Here's how the part is built. I have some questions about the finished solid (model axes, mm). A direction names the side the tool comes from. Give positions to 0.01 mm unless a question says otherwise; leave off trailing zeros. Write each loop counter-clockwise with the first axis right and the second up, starting at its lowest first coordinate (ties: lowest second). Pieces come first, ordered by that corner, then holes. Notation, with made-up numbers: (-26.5, 23) -> (-22.5, 23) arc R25 ccw to (-22.5, 59) -> close; hole circle Ø4 at (-4.75, -37). An arc over 180 degrees is marked (long way). Put each result on its own line as item: value. Start each with the question number.
from build123d import *

# Parameters (mm, degrees)
SKETCH_1_W      = 104
SKETCH_1_H      = 64
SKETCH_1_W_2    = 98
SKETCH_1_H_2    = 58
EXTRUDE_1_DEPTH = 2
SKETCH_1_3_W    = 104
SKETCH_1_3_H    = 64
EXTRUDE_2_DEPTH = 3
SKETCH_2_W      = 2
SKETCH_2_H      = 5
SKETCH_2_W_2    = 10
SKETCH_2_H_2    = 2
EXTRUDE_3_DEPTH = 2
EXTRUDE_START   = 2
SKETCH_1_4_W    = 104
SKETCH_1_4_H    = 64
SKETCH_1_4_W_2  = 98
SKETCH_1_4_H_2  = 58
EXTRUDE_4_DEPTH = 8.5
SKETCH_3_W      = 10
SKETCH_3_H      = 2
EXTRUDE_5_DEPTH = 2
EXTRUDE_START_2 = 10.5
SKETCH_1_5_W    = 104
SKETCH_1_5_H    = 64
SKETCH_1_5_W_2  = 98
SKETCH_1_5_H_2  = 58
EXTRUDE_6_DEPTH = 2


with BuildPart() as part:
    # 草图1 → 凸台-拉伸1 (new body)
    with BuildSketch(Plane(origin=(0, 0, 0), x_dir=(1, 0, 0), z_dir=(0, 1, 0))):
        Rectangle(SKETCH_1_W, SKETCH_1_H)
        Rectangle(SKETCH_1_W_2, SKETCH_1_H_2, mode=Mode.SUBTRACT)
    extrude(amount=EXTRUDE_1_DEPTH)

    # 草图1<3> → 凸台-拉伸2 (add)
    with BuildSketch(Plane(origin=(0, 0, 0), x_dir=(1, 0, 0), z_dir=(0, 1, 0))):
        Rectangle(SKETCH_1_3_W, SKETCH_1_3_H)
    extrude(amount=-EXTRUDE_2_DEPTH)

    # 草图2 → 凸台-拉伸3 (add)
    with BuildSketch(Plane(origin=(0, 0, 0), x_dir=(1, 0, 0), z_dir=(0, 1, 0))):
        with Locations((-48, 0)):
            Rectangle(SKETCH_2_W, SKETCH_2_H)
        with Locations((48, 0)):
            Rectangle(SKETCH_2_W, SKETCH_2_H)
        with Locations((0, 28)):
            Rectangle(SKETCH_2_W_2, SKETCH_2_H_2)
        with Locations((0, -28)):
            Rectangle(SKETCH_2_W_2, SKETCH_2_H_2)
    extrude(amount=EXTRUDE_3_DEPTH)

    # 草图1<4> → 凸台-拉伸4 (add)
    with BuildSketch(Plane(origin=(0, 0, 0), x_dir=(1, 0, 0), z_dir=(0, 1, 0)).offset(EXTRUDE_START)):
        Rectangle(SKETCH_1_4_W, SKETCH_1_4_H)
        Rectangle(SKETCH_1_4_W_2, SKETCH_1_4_H_2, mode=Mode.SUBTRACT)
    extrude(amount=EXTRUDE_4_DEPTH)

    # 草图3 → 凸台-拉伸5 (add)
    with BuildSketch(Plane(origin=(0, 10.5, 0), x_dir=(1, 0, 0), z_dir=(0, 1, 0))):
        with Locations((40, -28)):
            Rectangle(SKETCH_3_W, SKETCH_3_H)
        with Locations((-40, -28)):
            Rectangle(SKETCH_3_W, SKETCH_3_H)
        with Locations((40, 28)):
            Rectangle(SKETCH_3_W, SKETCH_3_H)
        with Locations((-40, 28)):
            Rectangle(SKETCH_3_W, SKETCH_3_H)
    extrude(amount=-EXTRUDE_5_DEPTH)

    # 草图1<5> → 凸台-拉伸6 (add)
    with BuildSketch(Plane(origin=(0, 0, 0), x_dir=(1, 0, 0), z_dir=(0, 1, 0)).offset(EXTRUDE_START_2)):
        Rectangle(SKETCH_1_5_W, SKETCH_1_5_H)
        Rectangle(SKETCH_1_5_W_2, SKETCH_1_5_H_2, mode=Mode.SUBTRACT)
    extrude(amount=EXTRUDE_6_DEPTH)


solid = part.part
1) Thinking about a two-plate mould opening in Y: for faces 1 (the flat face through (-48, 1, -2.5)), 2 (the flat face through (-1, 6, 29)), 3 (the flat face through (40, 8.5, 28)), 4 (the flat face through (-1, -3, 0)), which applies, released by +Y, released by -Y, zero draft, split by the parting line, or undercut?
2) I want a section at D-D, the plane x = -10. Write out the boundary of the cut face in (y, z), and give its area (3 significant figures).
3) I want a section at A-A, the plane x = 37.5. Write out the boundary of the cut face in (y, z).
4) I need wall thicknesses on probe 1 along X at (y, z) = (1.5, 10); probe 2 along Z at (x, y) = (48.5, 7.25); probe 3 along X at (y, z) = (10, 27.5). Which ranges of each line are inside material? Lowest first, please.
5) I want a section at C-C, the plane z = 18.5. Write out the boundary of the cut face in (x, y), and give its area (3 significant figures).
6) Which directions (+Z, -Z, +X, -X, +Y, -Y) give clear straight access to the entire face, cutting with the end or side of a thin tool? Please do faces 5 (the flat face through (52, 5, 0)), 6 (the flat face through (-40, 8.5, 28)), 7 (the flat face through (40, 10, -27)).
7) I'm going to push flat-ended pins straight in: pin 1 Ø3 at (x, z) = (35.5, 3.5) entering from +Y; pin 2 Ø0.6 at (x, z) = (-39, 28) entering from +Y. Where does each tip first touch, or does it pass through?
8) I want a section at B-B, the plane y = 4.25. Write out the boundary of the cut face in (x, z), and give its area (3 significant figures).
Established:
1. face 1: zero draft
1. face 2: undercut
1. face 3: undercut
1. face 4: released by -Y
2. outline: (-3, -32) -> (12.5, -32) -> (12.5, -29) -> (0, -29) -> (0, 29) -> (12.5, 29) -> (12.5, 32) -> (-3, 32) -> close
2. area: 267 mm2
3. outline: (-3, -32) -> (12.5, -32) -> (12.5, -29) -> (10.5, -29) -> (10.5, -27) -> (8.5, -27) -> (8.5, -29) -> (0, -29) -> (0, 29) -> (8.5, 29) -> (8.5, 27) -> (10.5, 27) -> (10.5, 29) -> (12.5, 29) -> (12.5, 32) -> (-3, 32) -> close
4. probe 1: x = -52 to -49, 49 to 52
4. probe 2: z = -32 to -29, 29 to 32
4. probe 3: x = -52 to -49, -45 to -35, 35 to 45, 49 to 52
5. outline: (-52, -3) -> (52, -3) -> (52, 12.5) -> (49, 12.5) -> (49, 0) -> (-49, 0) -> (-49, 12.5) -> (-52, 12.5) -> close
5. area: 387 mm2
6. face 5: +Z, -Z, +X, +Y, -Y
6. face 6: none
6. face 7: +Y
7. pin 1: stops at y = 0
7. pin 2: stops at y = 10.5
8. outline: (-52, -32) -> (52, -32) -> (52, 32) -> (-52, 32) -> close; hole (-49, -29) -> (49, -29) -> (49, 29) -> (-49, 29) -> close
8. area: 972 mm2
